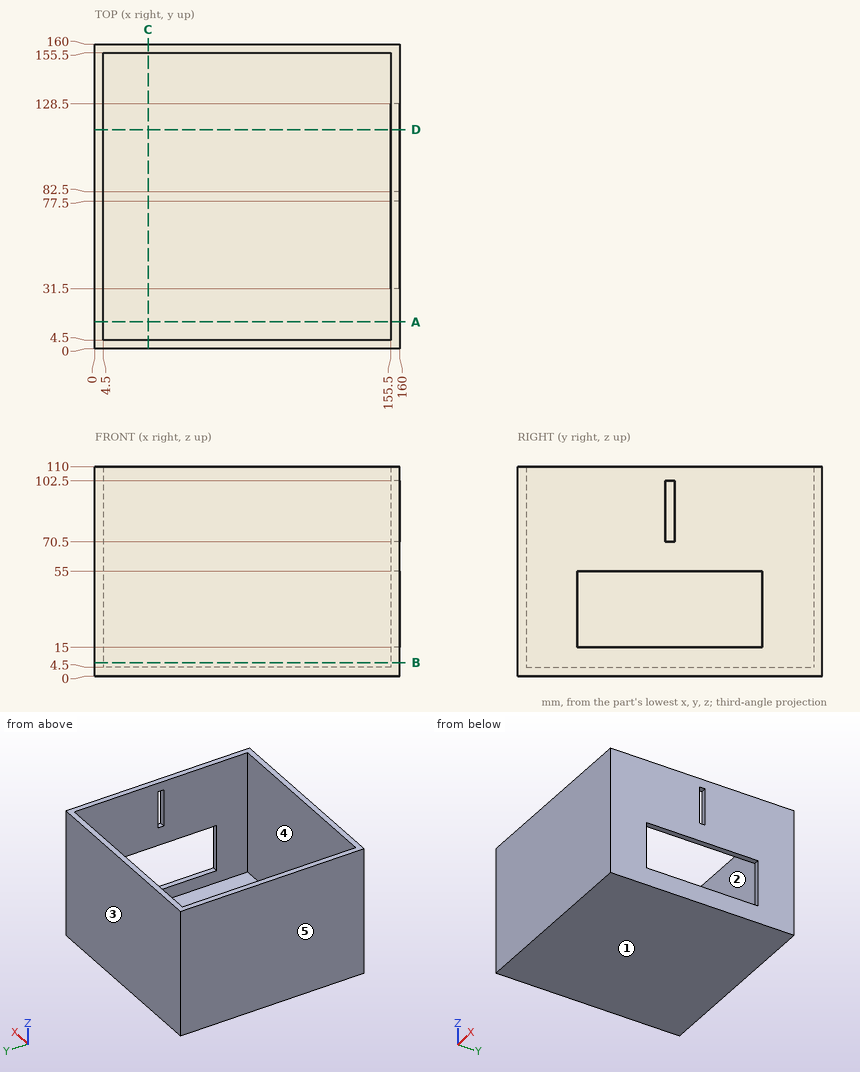
For this review, use the dimensioned drawing (mm, ordinates from the lowest corner) and the shaded views. A direction names the side the tool comes from. Round coordinates to 2 decimals unless told otherwise and drop trailing zeros. Order: outer loops, then holes, each group sorted by start corner. A loop starts at its lowest first (then second) coordinate and runs counter-clockwise, first axis right, second up. Notation, with made-up numbers: M 29.25,26.5 L 88.25,26.5 A31 cw 88.25,56.5 Z; hole C -19.75,22 d6. An arc over 180 degrees is marked long. Write each question's results on one line, items separated by ' | '. Start each with the question number.
1. Tool access review of the marked faces 1 and 2: name each direction out of +Z, -Z, +X, -X, +Y, -Y from which nothing blocks a thin tool from reaching the whole face with its end or side.
2. Add section D-D (y = 115). State the section outline as (x, z) points, then the cut area to 3 significant figures.
3. To check wall thickness, follow L1, parallel to X at y = 73, z = 7; L2, parallel to Z at x = 53, y = 24.5. State the ranges of each line that lie inside material, in increasing order. Write a range as [from, to].
4. Draft analysis for pull direction X (two halves, no side actions). For the marked faces 3, 4 and 5, state which applies: pulls with the +X half, pulls with the -X half, needs draft (parallel to the pull), parting line crosses it, or undercut.
5. Clearance check with a flat-ended pin moving along its axis: pin 1 Ø1.5 at (x, y) = (135, 105.5) entering from +Z. State where the tip first meets the part, or that it passes through.
6. Add section A-A (y = 14). State the section outline as (x, z) points.
7. Add section B-B (z = 7). State the section outline as (x, y) points.
Output values:
1) face 1: -Z, +X, -X, +Y, -Y | face 2: +Z
2) outline: M 0,0 L 160,0 L 160,15 L 155.5,15 L 155.5,4.5 L 4.5,4.5 L 4.5,110 L 0,110 Z; M 155.5,55 L 160,55 L 160,110 L 155.5,110 Z | area: 1,490 mm^2
3) L1: [0, 4.5], [155.5, 160] | L2: [0, 4.5]
4) face 3: needs draft | face 4: undercut | face 5: pulls with the -X half
5) pin 1: z = 4.5
6) outline: M 0,0 L 160,0 L 160,110 L 155.5,110 L 155.5,4.5 L 4.5,4.5 L 4.5,110 L 0,110 Z
7) outline: M 0,0 L 160,0 L 160,160 L 0,160 Z; hole M 4.5,4.5 L 155.5,4.5 L 155.5,155.5 L 4.5,155.5 Z
